Model file for the job. Use its own axes, mm. A direction names the side the tool comes from. Coordinates: 2 decimals unless noted, no trailing zeros. Write each loop counter-clockwise with the first axis right and the second up, starting at its lowest first coordinate (ties: lowest second). Pieces come first, ordered by that corner, then holes. Notation, with made-up numbers: (47, 50) - (75, 50) arc R5 cw to (75, 57) - close; hole circle Ø7 at (-7, 73.25). An arc over 180 degrees is marked (long way). Put each result on its own line as item: value. Start each with the question number.
1. Which spindle directions (+Z, -Z, +X, -X, +Y, -Y) get a long thin tool onto all of the face, cutting with end or side? Do faces 4 (the face through (16.9, -13.6, -1.6)), 5 (the face through (38.5, -19.5, 2.3)), 6 (the face through (2.688, 4.716, -0.944)). Say none if no direction does.
2. Saw through at D-D, the plane y = -1. Write the cut outline in (x, z), plus the area to 3 significant figures.
3. Drill centre lines: L1, parallel to Y at x = -15.5, z = 2; L2, parallel to X at y = 14.5, z = -2.5; L3, parallel to Y at x = 17, z = 0. Where is each one in solid material? Low to high. Write a range as from..to.
4. Saw through at A-A, the plane x = -42.5. Write the cut outline in (y, z).
5. Saw through at C-C, the plane x = 15.5. Write the cut outline in (y, z).
6. Saw through at B-B, the plane z = -4. Give the number of separate pieces and of enclosed holes in the cut face, plus the area to 3 significant figures.
7. Pull direction Y, two halves, no side cores. Call faces 1 (the face through (50, -10, 0)), 2 (the face through (39.9, 12.6, 0.1)), 3 (the face through (-15.923, 12.778, -3.324)): released by +Y, released by -Y, zero draft, split by the parting line, or undercut.
8. Drop flat-ended pins along their axis: P1, Ø6.5, axis at x = -42.5, y = -16.5, coming from the +Z side; P2, Ø2, axis at x = -15.5, y = -16, coming from the -Z side; P3, Ø1.5, axis at x = -32, z = -3, coming from the +Y side; P4, Ø6, axis at x = 0, y = 0.5, coming from the -Z side. Give the stop position or say it passes through.
```python
from build123d import *

# Parameters (mm, degrees)
SKETCH1_W                                           = 100
SKETCH1_H                                           = 45
BOSS_EXTRUDE1_DEPTH                                 = 5
CHAMFER1_SIZE                                       = 20
CBORE_FOR_M5_HEX_SOCKET_HEAD_CAP_SCREW2_D           = 5.5
CBORE_FOR_M5_HEX_SOCKET_HEAD_CAP_SCREW2_CBORE_D     = 10
CBORE_FOR_M5_HEX_SOCKET_HEAD_CAP_SCREW2_CBORE_DEPTH = 5.4
CBORE_FOR_M3_HEX_SOCKET_HEAD_CAP_SCREW1_D           = 3.4
CBORE_FOR_M3_HEX_SOCKET_HEAD_CAP_SCREW1_CBORE_D     = 6.5
CBORE_FOR_M3_HEX_SOCKET_HEAD_CAP_SCREW1_CBORE_DEPTH = 3.4
SKETCH2_R                                           = 5
CUT_EXTRUDE3_DEPTH                                  = 10
SKETCH12_R                                          = 11.25
CUT_EXTRUDE4_DEPTH                                  = 2


with BuildPart() as part:
    # Sketch1 → Boss-Extrude1 (new, symmetric)
    with BuildSketch(Plane.XY):
        Rectangle(SKETCH1_W, SKETCH1_H)
    extrude(amount=BOSS_EXTRUDE1_DEPTH, both=True)

    # Chamfer1
    chamfer1_edges = [part.edges().sort_by_distance(p)[0] for p in [
        (-50, 22.5, 0),
        (50, 22.5, 0),
    ]]
    chamfer(chamfer1_edges, length=CHAMFER1_SIZE)

    # CBORE for M5 Hex Socket Head Cap Screw2 (through all)
    with Locations(Plane.XY.offset(5)):
        with Locations((-42.5, -16.5), (-27.5, -16.5), (27.5, -16.5), (42.5, -16.5)):
            CounterBoreHole(CBORE_FOR_M5_HEX_SOCKET_HEAD_CAP_SCREW2_D / 2, CBORE_FOR_M5_HEX_SOCKET_HEAD_CAP_SCREW2_CBORE_D / 2, CBORE_FOR_M5_HEX_SOCKET_HEAD_CAP_SCREW2_CBORE_DEPTH)

    # CBORE for M3 Hex Socket Head Cap Screw1 (through all)
    with Locations(Plane(origin=(0, 0, -5), x_dir=(1, 0, 0), z_dir=(0, 0, -1))):
        with Locations((-15.5, -16), (15.5, -16), (15.5, 15), (-15.5, 15)):
            CounterBoreHole(CBORE_FOR_M3_HEX_SOCKET_HEAD_CAP_SCREW1_D / 2, CBORE_FOR_M3_HEX_SOCKET_HEAD_CAP_SCREW1_CBORE_D / 2, CBORE_FOR_M3_HEX_SOCKET_HEAD_CAP_SCREW1_CBORE_DEPTH)

    # Sketch2 → Cut-Extrude3 (cut)
    with BuildSketch(Plane.XY.offset(5)):
        with Locations((0, 0.5)):
            Circle(SKETCH2_R)
    extrude(amount=-CUT_EXTRUDE3_DEPTH, mode=Mode.SUBTRACT)

    # Sketch12 → Cut-Extrude4 (cut)
    with BuildSketch(Plane(origin=(0, 0, 5), x_dir=(-1, 0, 0), z_dir=(0, 0, -1))):
        Circle(SKETCH12_R)
    extrude(amount=CUT_EXTRUDE4_DEPTH, mode=Mode.SUBTRACT)


solid = part.part
```
Final values:
1. face 4: -Z
1. face 5: +Z
1. face 6: +Z, -Z
2. outline: (-50, -5) - (-4.77, -5) - (-4.77, 3) - (-11.21, 3) - (-11.21, 5) - (-50, 5) - close; (4.77, -5) - (50, -5) - (50, 5) - (11.21, 5) - (11.21, 3) - (4.77, 3) - close
2. area: 879 mm²
3. L1: y = -22.5..-16.7, -13.3..14.3, 17.7..22.5
3. L2: x = -38..-18.38, -12.62..12.62, 18.38..38
3. L3: y = -22.5..-15.8, -14.2..15.2, 16.8..22.5
4. outline: (-22.5, -5) - (-19.25, -5) - (-19.25, -0.4) - (-21.5, -0.4) - (-21.5, 5) - (-22.5, 5) - close; (-13.75, -5) - (10, -5) - (10, 5) - (-11.5, 5) - (-11.5, -0.4) - (-13.75, -0.4) - close
5. outline: (-22.5, -5) - (-18.25, -5) - (-18.25, -1.6) - (-16.7, -1.6) - (-16.7, 5) - (-22.5, 5) - close; (-13.3, -1.6) - (-11.75, -1.6) - (-11.75, -5) - (12.75, -5) - (12.75, -1.6) - (14.3, -1.6) - (14.3, 5) - (-13.3, 5) - close; (17.7, -1.6) - (19.25, -1.6) - (19.25, -5) - (22.5, -5) - (22.5, 5) - (17.7, 5) - close
6. separate pieces: 1
6. enclosed holes: 9
6. area: 3,790 mm²
7. face 1: zero draft
7. face 2: released by +Y
7. face 3: undercut
8. P1: stops at z = -0.4
8. P2: stops at z = -1.6
8. P3: stops at y = 21.25
8. P4: passes through
